Can you work these out from the model? Positions are in its coordinate system, mm. A direction names the side the tool comes from. Round coordinates to 2 decimals unless told otherwise and drop trailing zeros. Loops run counter-clockwise (first coordinate to the right, second up) from the corner with the lowest first, then second, coordinate; pieces in that order, holes last. Notation, with made-up numbers: (-23.75, 2) -> (35.25, 2) arc R22 cw to (35.25, 41) -> close; hole circle Ø6 at (4.5, 51). An arc over 180 degrees is marked (long way). Write item = value, one per line.
from build123d import *
from build123d.topology import SkipClean

# Parameters (mm, degrees)
BOSS_EXTRUDE1_REACH     = 80.339
CUT_EXTRUDE1_DEPTH      = 87.068697729
CUT_EXTRUDE1_DEPTH_BACK = 87.068697729
GUDGEON_HOLE_R          = 15
CUT_EXTRUDE2_DEPTH      = 103.318131503
RING_CS_W               = 2
RING_CS_H               = 1
BOSS_EXTRUDE2_DEPTH     = 3
FILLET1_R               = 3


with BuildPart() as part:
    # Piston CS → Revolve1 (revolve)
    with BuildSketch(Plane.XY, mode=Mode.PRIVATE) as revolve1_sk:
        Polygon((0, 0), (0, -5), (27, -5), (30, -6.732050808), (30, -16.732050808), (35, -16.732050808), (35, -57), (38, -57), (38, -5), (37, -5), (28.339745962, 0), align=None)
    revolve(revolve1_sk.sketch.rotate(Axis((0, 0, 0), (0, -1, 0)), 90), axis=Axis((0, 0, 0), (0, -1, 0)))

    # Sketch5 → Boss-Extrude1 (add, up to next)
    with BuildSketch(Plane.XZ.offset(57), mode=Mode.PRIVATE) as boss_extrude1_sk1:
        with BuildLine():
            Line((-24.103941586, -38), (-24.103941586, -18))
            Line((-24.103941586, -18), (-14.103941586, -18))
            Line((-14.103941586, -18), (-14.103941586, 18))
            Line((-14.103941586, 18), (-24.103941586, 18))
            Line((-24.103941586, 18), (-24.103941586, 38))
            ThreePointArc((-24.103941586, 38), (-45, 0), (-24.103941586, -38))
        make_face()
    boss_extrude1_tool1 = extrude(boss_extrude1_sk1.sketch, amount=-BOSS_EXTRUDE1_REACH, mode=Mode.PRIVATE) - part.part
    # Sketch5 → Boss-Extrude1 (add, up to next)
    with BuildSketch(Plane.XZ.offset(57), mode=Mode.PRIVATE) as boss_extrude1_sk2:
        with BuildLine():
            Line((24.103941586, 38), (24.103941586, 18))
            Line((24.103941586, 18), (14.103941586, 18))
            Line((14.103941586, 18), (14.103941586, -18))
            Line((14.103941586, -18), (24.103941586, -18))
            Line((24.103941586, -18), (24.103941586, -38))
            ThreePointArc((24.103941586, -38), (45, 0), (24.103941586, 38))
        make_face()
    boss_extrude1_tool2 = extrude(boss_extrude1_sk2.sketch, amount=-BOSS_EXTRUDE1_REACH, mode=Mode.PRIVATE) - part.part
    add(boss_extrude1_tool1.solids().sort_by_distance((-29.359208, -57, 0))[0])
    add(boss_extrude1_tool2.solids().sort_by_distance((29.359208, -57, 0))[0])

    # Gudgeon Hole → Cut-Extrude1 (cut, two sides: drawn at the far end of the back side and taken through both)
    with BuildSketch(Plane(origin=(-14.103941586, 0, 0), x_dir=(0, 0, -1), z_dir=(1, 0, 0)).offset(-CUT_EXTRUDE1_DEPTH_BACK)):
        with Locations((0, -27)):
            Circle(GUDGEON_HOLE_R)
    extrude(amount=CUT_EXTRUDE1_DEPTH + CUT_EXTRUDE1_DEPTH_BACK, mode=Mode.SUBTRACT)

    # Gudgeon Hole Cutouts → Cut-Extrude2 (cut, through all)
    with BuildSketch(Plane.XY.offset(38)):
        with BuildLine():
            Line((33.9141805, -12), (33.9141805, -42))
            Line((33.9141805, -42), (38, -42))
            add(Edge.make_bspline(
                [(38, -42), (32.078947368, -27), (38, -12)],
                knots=[0, 0, 0, 1, 1, 1], degree=2, weights=[0.023, 0.038, 0.053]))
            Line((38, -12), (33.9141805, -12))
        make_face()
        with BuildLine():
            Line((-38, -12), (-33.9141805, -12))
            Line((-33.9141805, -12), (-33.9141805, -42))
            Line((-33.9141805, -42), (-38, -42))
            add(Edge.make_bspline(
                [(-38, -12), (-32.078947368, -27), (-38, -42)],
                knots=[0, 0, 0, 1, 1, 1], degree=2, weights=[0.023, 0.038, 0.053]))
        make_face()
    extrude(amount=-CUT_EXTRUDE2_DEPTH, mode=Mode.SUBTRACT)

    # Ring CS → Cut-Revolve1 (revolve, cut)
    with BuildSketch(Plane.XY, mode=Mode.PRIVATE) as cut_revolve1_sk:
        with Locations((37, -6.5)):
            Rectangle(RING_CS_W, RING_CS_H)
        with Locations((37, -9.5)):
            Rectangle(RING_CS_W, RING_CS_H)
    revolve(cut_revolve1_sk.sketch.rotate(Axis((0, 0, 0), (0, -1, 0)), 90), axis=Axis((0, 0, 0), (0, -1, 0)), mode=Mode.SUBTRACT)

    # Sketch9 → Boss-Extrude2 (add)
    with SkipClean():  # the faces are left unmerged after this step: merging them gives an invalid solid
        with BuildSketch(Plane.XZ.offset(57)):
            with BuildLine():
                Line((-1.526678558, 34.966687755), (-1.65753672, 37.96383242))
                ThreePointArc((-1.65753672, 37.96383242), (0, 38), (1.65753672, 37.96383242))
                Line((1.65753672, 37.96383242), (1.526678558, 34.966687755))
                ThreePointArc((1.526678558, 34.966687755), (0, 35), (-1.526678558, 34.966687755))
            make_face()
            with BuildLine():
                Line((1.526678558, -34.966687755), (1.65753672, -37.96383242))
                ThreePointArc((1.65753672, -37.96383242), (0, -38), (-1.65753672, -37.96383242))
                Line((-1.65753672, -37.96383242), (-1.526678558, -34.966687755))
                ThreePointArc((-1.526678558, -34.966687755), (0, -35), (1.526678558, -34.966687755))
            make_face()
        extrude(amount=BOSS_EXTRUDE2_DEPTH)

    # Fillet1
    # the kernel refuses this fillet: 3 mm, written as the material it adds along each edge
    with BuildSketch(Plane(origin=(1.984682125, -57, 45.456694082), x_dir=(0.9990482215818575, 0, -0.04361938736534301), z_dir=(-0.043619387365343, 0, -0.9990482215818575))) as fillet1_piece_1_section:
        with BuildLine():
            CenterArc((FILLET1_R, FILLET1_R), FILLET1_R, 180, 90)
            Line((0, FILLET1_R), (0, 0))
            Line((0, 0), (FILLET1_R, 0))
        make_face()
    fillet1_piece_1 = extrude(amount=18, mode=Mode.PRIVATE)
    fillet1_piece_1 = fillet1_piece_1 & Plane(origin=(0, -57.679016135, 0), x_dir=(0, 0, 1), z_dir=(0, 1, 0)) * Cylinder(38, 49, mode=Mode.PRIVATE)
    fillet1_piece_1 = fillet1_piece_1 - Plane(origin=(0, -57.679016135, 0), x_dir=(0, 0, 1), z_dir=(0, -1, 0)) * Cylinder(35, 49, mode=Mode.PRIVATE)
    add(fillet1_piece_1)
    with BuildSketch(Plane(origin=(-1.199533153, -57, 27.473826094), x_dir=(-0.999048221581858, 0, -0.04361938736532912), z_dir=(-0.043619387365329124, 0, 0.9990482215818581))) as fillet1_piece_2_section:
        with BuildLine():
            CenterArc((FILLET1_R, FILLET1_R), FILLET1_R, 180, 90)
            Line((0, FILLET1_R), (0, 0))
            Line((0, 0), (FILLET1_R, 0))
        make_face()
    fillet1_piece_2 = extrude(amount=18, mode=Mode.PRIVATE)
    fillet1_piece_2 = fillet1_piece_2 & Plane(origin=(0, -57.679023016, 0), x_dir=(0, 0, 1), z_dir=(0, 1, 0)) * Cylinder(38, 48, mode=Mode.PRIVATE)
    fillet1_piece_2 = fillet1_piece_2 - Plane(origin=(0, -57.679023016, 0), x_dir=(0, 0, 1), z_dir=(0, -1, 0)) * Cylinder(35, 48, mode=Mode.PRIVATE)
    add(fillet1_piece_2)
    with BuildSketch(Plane(origin=(1.199533153, -57, -27.473826094), x_dir=(0.9990482215818575, 0, 0.043619387365343), z_dir=(0.043619387365343, 0, -0.9990482215818575))) as fillet1_piece_3_section:
        with BuildLine():
            CenterArc((FILLET1_R, FILLET1_R), FILLET1_R, 180, 90)
            Line((0, FILLET1_R), (0, 0))
            Line((0, 0), (FILLET1_R, 0))
        make_face()
    fillet1_piece_3 = extrude(amount=18, mode=Mode.PRIVATE)
    fillet1_piece_3 = fillet1_piece_3 & Plane(origin=(0, -57.679021067, 0), x_dir=(0, 0, 1), z_dir=(0, 1, 0)) * Cylinder(38, 49, mode=Mode.PRIVATE)
    fillet1_piece_3 = fillet1_piece_3 - Plane(origin=(0, -57.679021067, 0), x_dir=(0, 0, 1), z_dir=(0, -1, 0)) * Cylinder(35, 49, mode=Mode.PRIVATE)
    add(fillet1_piece_3)
    with BuildSketch(Plane(origin=(-1.984682125, -57, -45.456694082), x_dir=(-0.999048221581858, 0, 0.04361938736532913), z_dir=(0.043619387365329124, 0, 0.9990482215818581))) as fillet1_piece_4_section:
        with BuildLine():
            CenterArc((FILLET1_R, FILLET1_R), FILLET1_R, 180, 90)
            Line((0, FILLET1_R), (0, 0))
            Line((0, 0), (FILLET1_R, 0))
        make_face()
    fillet1_piece_4 = extrude(amount=18, mode=Mode.PRIVATE)
    fillet1_piece_4 = fillet1_piece_4 - Plane(origin=(0, -57.679020805, 0), x_dir=(0, 0, 1), z_dir=(0, -1, 0)) * Cylinder(35, 48, mode=Mode.PRIVATE)
    fillet1_piece_4 = fillet1_piece_4 & Plane(origin=(0, -57.679020805, 0), x_dir=(0, 0, 1), z_dir=(0, 1, 0)) * Cylinder(38, 48, mode=Mode.PRIVATE)
    add(fillet1_piece_4)


solid = part.part
1. Suppose I cut it at B-B, the plane y = -53. List the corners of the cut face in (x, z) for me, and give its area (3 significant figures).
Entries:
outline = circle Ø76 at (0, 0); hole (-24.1, -25.38) arc R35 ccw to (24.1, -25.38) -> (24.1, -18) -> (14.1, -18) -> (14.1, 18) -> (24.1, 18) -> (24.1, 25.38) arc R35 ccw to (-24.1, 25.38) -> (-24.1, 18) -> (-14.1, 18) -> (-14.1, -18) -> (-24.1, -18) -> close
area = 2,170 mm²
2. Suppose I cut it at D-D, the plane z = -3.5. Count the separate pieces of the cut face and the enclosed holes in it, and give its area (3 significant figures).
Entries:
separate_pieces = 3
enclosed_holes = 0
area = 1,390 mm²
3. I'm going to push flat-ended pins straight in: pin 1 (1.2 mm diameter, centred on x = -35.5, z = -3, fed in from -Y); pin 2 (8.5 mm diameter, centred on y = -31.5, z = -12, fed in from +X); pin 3 (12 mm diameter, centred on y = -51, z = 5, fed in from +X); pin 4 (3 mm diameter, centred on x = -26, z = -15, fed in from +Y). Where does each tip first touch, or does it pass through?
Entries:
pin_1 = -57
pin_2 = 33.91
pin_3 = 38
pin_4 = -0.1
4. For faces 4 (the flat face through (33.914, -26, 16)), 5 (the cylindrical face through (-24.331, -9.493, -26.533)), 6 (the flat face through (24.104, -37, 22)), which set-ups out of +Z, -Z, +X, -X, +Y, -Y let a thin tool reach every point of the face, with its end or its side?
Entries:
face_4 = +Z, -Z, +X
face_5 = none
face_6 = -Y
5. Suppose I cut it at A-A, the plane y = -27. List the corners of the cut face in (x, z) for me, and give its area (3 significant figures).
Entries:
outline = (-33.91, -17.14) arc R38 ccw to (33.91, -17.14) -> (33.91, -15) -> (14.1, -15) -> (14.1, -18) -> (24.1, -18) -> (24.1, -25.38) arc R35 cw to (-24.1, -25.38) -> (-24.1, -18) -> (-14.1, -18) -> (-14.1, -15) -> (-33.91, -15) -> close; (-33.91, 15) -> (-14.1, 15) -> (-14.1, 18) -> (-24.1, 18) -> (-24.1, 25.38) arc R35 cw to (24.1, 25.38) -> (24.1, 18) -> (14.1, 18) -> (14.1, 15) -> (33.91, 15) -> (33.91, 17.14) arc R38 ccw to (-33.91, 17.14) -> close
area = 794 mm²
6. We'd pull the mould along X, two halves only. Please class faces 1 (the cylindrical face through (2.443, -57.902, -36.342)), 2 (the cylindrical face through (0, -12, 30)), 3 (the flat face through (36, -12, 0)): released by +X, released by -X, zero draft, split by the parting line, or undercut.
Entries:
face_1 = released by +X
face_2 = undercut
face_3 = zero draft
7. I need wall thicknesses on line 1 (Z direction, x = 21, y = -27); line 2 (Z direction, x = -15, y = -40.5); line 3 (Y direction, x = -27.5, z = 0). Which ranges of each line are inside material? Lowest first, please. Write a range as [from, to].
Entries:
line_1 = [-31.67, -28], [-18, -15], [15, 18], [28, 31.67]
line_2 = [-34.91, -31.62], [-18, -6.54], [6.54, 18], [31.62, 34.91]
line_3 = [-57, -42], [-12, 0]
